Model file for the job. Use its own axes, mm. Face numbers are marked on the shaded views. A direction names the side the tool comes from. Round coordinates to 2 decimals unless told otherwise and drop trailing zeros. Loops run counter-clockwise (first coordinate to the right, second up) from the corner with the lowest first, then second, coordinate; pieces in that order, holes last. Notation, with made-up numbers: (87, -14) - (145, -14) arc R11 ccw to (145, -8) - close; hole circle Ø8 at (58.5, 41.25). An arc over 180 degrees is marked (long way). Answer as a JSON object with one key per item and string values.
from build123d import *

# Parameters (mm, degrees)
SKETCH1_R           = 22
BOSS_EXTRUDE1_DEPTH = 36
SKETCH3_R           = 19.375
CUT_EXTRUDE1_DEPTH  = 33.25
SKETCH4_W           = 13
SKETCH4_H           = 8.241634072
CUT_EXTRUDE2_DEPTH  = 33.25
SKETCH5_R           = 3.175
BOSS_EXTRUDE2_DEPTH = 7


with BuildPart() as part:
    # Sketch1 → Boss-Extrude1 (new body)
    with BuildSketch(Plane(origin=(0, 0, 0), x_dir=(1, 0, 0), z_dir=(0, 1, 0))):
        Circle(SKETCH1_R)
    extrude(amount=BOSS_EXTRUDE1_DEPTH)

    # Sketch3 → Cut-Extrude1 (cut)
    with BuildSketch(Plane(origin=(0, 36, 0), x_dir=(1, 0, 0), z_dir=(0, 1, 0))):
        Circle(SKETCH3_R)
    extrude(amount=-CUT_EXTRUDE1_DEPTH, mode=Mode.SUBTRACT)

    # Sketch4 → Cut-Extrude2 (cut)
    with BuildSketch(Plane(origin=(0, 36, 0), x_dir=(1, 0, 0), z_dir=(0, 1, 0))):
        with Locations((0, -20.83301946)):
            Rectangle(SKETCH4_W, SKETCH4_H)
    extrude(amount=-CUT_EXTRUDE2_DEPTH, mode=Mode.SUBTRACT)

    # Sketch5 → Boss-Extrude2 (add)
    with BuildSketch(Plane(origin=(0, 0, 0), x_dir=(-1, 0, 0), z_dir=(0, -1, 0))):
        with Locations((12.386484202, -12.411737756)):
            Circle(SKETCH5_R)
        with Locations((-12.413515798, -12.411737756)):
            Circle(SKETCH5_R)
        with Locations((-12.413515798, 12.388262244)):
            Circle(SKETCH5_R)
        with Locations((12.386484202, 12.388262244)):
            Circle(SKETCH5_R)
    extrude(amount=BOSS_EXTRUDE2_DEPTH)


solid = part.part
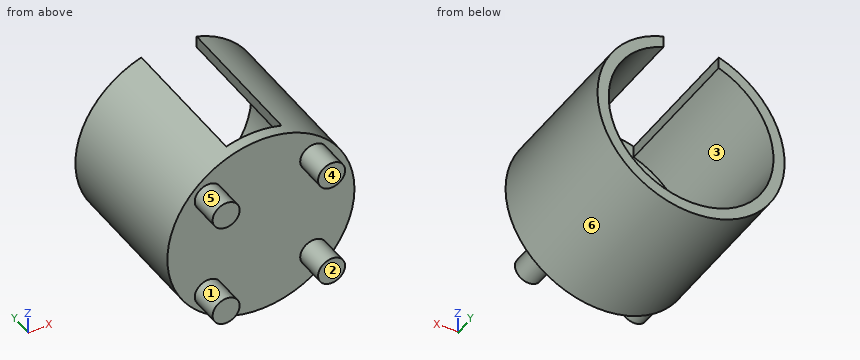
1) Tool access for the marked faces 1, 2 and 3: list every direction of +Z, -Z, +X, -X, +Y, -Y with a clear straight run to the whole face (end or side of a thin tool).
Values follow:
{"face 1": "-Y", "face 2": "+Z, -Z, +X, -X, -Y", "face 3": "+Y"}
2) Slice it at D-D on y = 11. List the corners of the cut face in (x, z) (3 decimals), then the cut area to 3 significant figures.
Values follow:
{"outline": "(-6.5, 18.252) - (-6.5, 21.018) arc R22 ccw (long way) to (6.5, 21.018) - (6.5, 18.252) arc R19.375 cw (long way) to start", "area": "306 mm²"}
3) Slice it at C-C on y = -3. List the corners of the cut face in (x, z) (3 decimals), then the cut area to 3 significant figures.
Values follow:
{"outline": "circle Ø6.35 at (-12.386, -12.388); circle Ø6.35 at (-12.386, 12.412); circle Ø6.35 at (12.414, -12.388); circle Ø6.35 at (12.414, 12.412)", "area": "127 mm²"}
4) Slice it at A-A on z = 0. List the corners of the cut face in (x, y) (3 decimals).
Values follow:
{"outline": "(-22, 0) - (22, 0) - (22, 36) - (19.375, 36) - (19.375, 2.75) - (-19.375, 2.75) - (-19.375, 36) - (-22, 36) - close"}
5) Probe probe 1 along X at (y, z) = (15, 0) (3 decimals); probe 2 along Z at (x, y) = (7, 13); probe 3 along Y at (x, z) = (17, 13). List the from-to ranges inside material, lowest first.
Values follow:
{"probe 1": "-22 to -19.375, 19.375 to 22", "probe 2": "-20.86 to -18.07, 18.07 to 20.86", "probe 3": "0 to 36"}
6) Drop flat-ended pins along their axis: P1, Ø1, axis at x = 6, z = -2.5, coming from the -Y side; P2, Ø10, axis at x = -16, y = 17, coming from the +Z side; P3, Ø1.4, axis at y = 21.5, z = 19.5, coming from the +X side. Give the stop position or say it passes through.
Values follow:
{"P1": "y = 0", "P2": "z = 19.05", "P3": "x = 11.43"}
7) Slice it at B-B on x = -12.5. List the corners of the cut face in (y, z).
Values follow:
{"outline": "(-7, -15.56) - (0, -15.56) - (0, -18.1) - (36, -18.1) - (36, -14.8) - (2.75, -14.8) - (2.75, 14.8) - (36, 14.8) - (36, 18.1) - (0, 18.1) - (0, 15.58) - (-7, 15.58) - (-7, 9.24) - (0, 9.24) - (0, -9.22) - (-7, -9.22) - close"}
8) Two-plate mould, pull along Z, no slides. Class the marked faces 4, 5 and 6: pulls with the +Z half, pulls with the -Z half, needs draft (parallel to the pull), parting line crosses it, or undercut.
Values follow:
{"face 4": "needs draft", "face 5": "undercut", "face 6": "parting line crosses it"}
